Geometry check sheet. Reference: the model listing, model coordinates, mm. Face numbers are marked on the shaded views. Give positions to 0.01 mm unless a question says otherwise; leave off trailing zeros. Order: outer loops, then holes, each group sorted by start corner. A loop starts at its lowest first (then second) coordinate and runs counter-clockwise, first axis right, second up.
from build123d import *

# Parameters (mm, degrees)
F0_W     = 75
F0_H     = 65
F1_DEPTH = 10
F3_D     = 14.5
F5_D     = 5


with BuildPart() as f1:
    # F0 (on Front) → F1 (new body)
    with BuildSketch(Plane.XZ):
        with Locations((37.5, 32.5)):
            Rectangle(F0_W, F0_H)
    extrude(amount=F1_DEPTH)

    # F3 (through all)
    with Locations(Plane.XZ.offset(10)):
        with Locations((37.950881, 48.491641), (37.950881, 22.491641)):
            Hole(F3_D / 2)

    # F5 (through all)
    with Locations(Plane.XZ.offset(10)):
        with Locations((16.265364, 53.577758), (16.952468, 40.109664), (61.576582, 25.720431), (61.264336, 14.315818)):
            Hole(F5_D / 2)


solid = f1.part
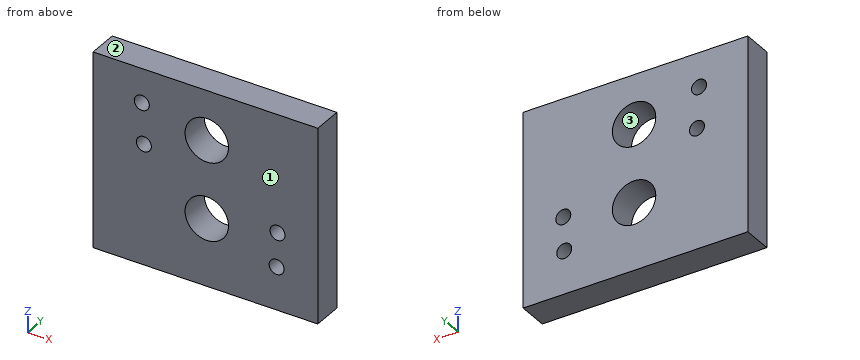
Item 1: Scan lines: L1, parallel to Z at x = 42, y = -2.25; L2, parallel to Z at x = 40, y = -7.75; L3, parallel to X at y = -9.5, z = 22.5. Record each from-to range of solid material in increasing order.
Reported:
L1: z = 0 to 16.48, 28.51 to 42.48, 54.51 to 65
L2: z = 0 to 15.54, 29.45 to 41.54, 55.45 to 65
L3: x = 0 to 30.7, 45.2 to 75
Item 2: Draft check along Z on the marked faces 1, 2 and 3. Enter one of: released by +Z, released by -Z, zero draft, split by the parting line, or undercut.
Reported:
face 1: zero draft
face 2: released by +Z
face 3: undercut
Item 3: Sectioned sample at A-A (z = 44). Enter the section's corners in (x, y).
Reported:
outline: (0, -10) - (32.26, -10) - (32.26, 0) - (0, 0) - close; (43.64, -10) - (75, -10) - (75, 0) - (43.64, 0) - close
Item 4: Sectioned sample at B-B (x = 37.5). Enter the section's corners in (y, z).
Reported:
outline: (-10, 0) - (0, 0) - (0, 15.26) - (-10, 15.26) - close; (-10, 29.73) - (0, 29.73) - (0, 41.26) - (-10, 41.26) - close; (-10, 55.73) - (0, 55.73) - (0, 65) - (-10, 65) - close
Item 5: Gauge pin test, flat end, axial feed: pin 1 (4.5 mm diameter, centred on x = 61.58, z = 25.72, fed in from +Y). Record the tip position at first contact, or that the pin passes through.
Reported:
pin 1: passes through
Item 6: Sectioned sample at C-C (y = -4.75). Enter the section's corners in (x, z), and give its area (3 significant figures).
Reported:
outline: (0, 0) - (75, 0) - (75, 65) - (0, 65) - close; hole circle Ø5 at (16.27, 53.58); hole circle Ø5 at (16.95, 40.11); hole circle Ø14.5 at (37.95, 22.49); hole circle Ø14.5 at (37.95, 48.49); hole circle Ø5 at (61.26, 14.32); hole circle Ø5 at (61.58, 25.72)
area: 4,470 mm2
